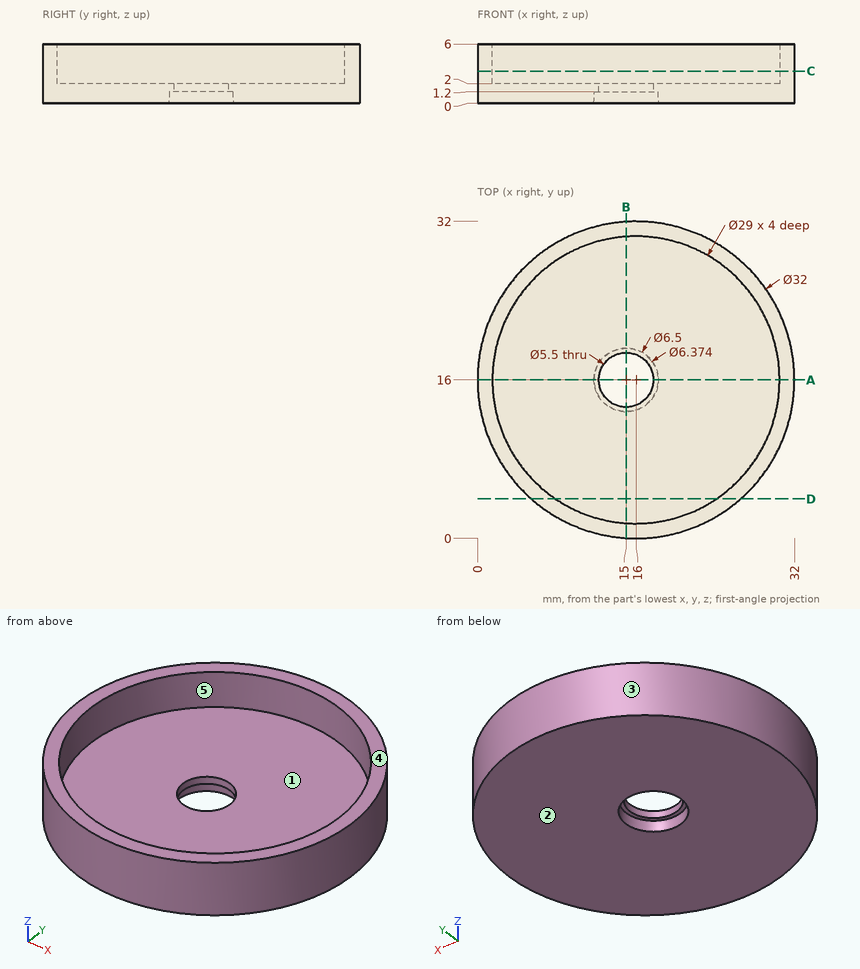
Print and shaded views of the part. All mm, measured from the part's lowest x, y and z. A direction names the side the tool comes from. Round coordinates to 2 decimals unless told otherwise and drop trailing zeros. Write each loop counter-clockwise with the first axis right and the second up, starting at its lowest first coordinate (ties: lowest second). Pieces come first, ordered by that corner, then holes. Notation, with made-up numbers: (75, 49.5) -> (93, 49.5) arc R24 cw to (93, 82.5) -> close; hole circle Ø11 at (-30, 53.25). An arc over 180 degrees is marked (long way). Answer in a Markdown table with one row per item. Add a question column.
Item 1: Drill centre lines: line 1 (Y direction, x = 16, z = 2.85); line 2 (Z direction, x = 22, y = 29); line 3 (X direction, y = 15, z = 0.95). Where is each one in solid material? Low to high. Write a range as from..to.
Item 2: Saw through at A-A, the plane y = 16. Write the cut outline in (x, z).
Item 3: Which spindle directions (+Z, -Z, +X, -X, +Y, -Y) get a long thin tool onto all of the face, cutting with end or side? Do the marked faces 4 and 5. Say none if no direction does.
Item 4: Drop flat-ended pins along their axis: pin 1 Ø12 at (x, y) = (5, 25) entering from +Z; pin 2 Ø1 at (x, y) = (14.5, 15) entering from -Z (3 decimals); pin 3 Ø1 at (x, z) = (26.5, 1) entering from +Y; pin 4 Ø1 at (x, y) = (16.5, 9.5) entering from +Z. Give the stop position or say it passes through.
Item 5: Mould opens along Y. For the marked faces 1, 2 and 3 say: pulls with the +Y half, pulls with the -Y half, needs draft (parallel to the pull), parting line crosses it, or undercut.
Item 6: Saw through at D-D, the plane y = 4. Write the cut outline in (x, z).
Item 7: Saw through at C-C, the plane z = 3.25. Write the cut outline in (x, y), then the cut area to 3 significant figures.
Item 8: Saw through at B-B, the plane x = 15. Write the cut outline in (y, z).
Findings below:
| question | item | result |
|---|---|---|
| 1 | line 1 | y = 0..1.5, 30.5..32 |
| 1 | line 2 | z = 0..2 |
| 1 | line 3 | x = 0.03..11.96, 18.04..31.97 |
| 2 | outline | (0, 0) -> (11.75, 0) -> (11.81, 1.2) -> (12.25, 1.2) -> (12.25, 2) -> (1.5, 2) -> (1.5, 6) -> (0, 6) -> close; (17.75, 1.2) -> (18.19, 1.2) -> (18.25, 0) -> (32, 0) -> (32, 6) -> (30.5, 6) -> (30.5, 2) -> (17.75, 2) -> close |
| 3 | face 4 | +Z, +X, -X, +Y, -Y |
| 3 | face 5 | +Z |
| 4 | pin 1 | stops at z = 6 |
| 4 | pin 2 | passes through |
| 4 | pin 3 | stops at y = 28.49 |
| 4 | pin 4 | stops at z = 2 |
| 5 | face 1 | undercut |
| 5 | face 2 | needs draft |
| 5 | face 3 | parting line crosses it |
| 6 | outline | (5.42, 0) -> (26.58, 0) -> (26.58, 6) -> (24.14, 6) -> (24.14, 2) -> (7.86, 2) -> (7.86, 6) -> (5.42, 6) -> close |
| 7 | outline | circle Ø32 at (16, 16); hole circle Ø29 at (16, 16) |
| 7 | area | 144 mm^2 |
| 8 | outline | (0.03, 0) -> (12.75, 0) -> (12.81, 1.2) -> (13.25, 1.2) -> (13.25, 2) -> (1.53, 2) -> (1.53, 6) -> (0.03, 6) -> close; (18.75, 1.2) -> (19.19, 1.2) -> (19.25, 0) -> (31.97, 0) -> (31.97, 6) -> (30.47, 6) -> (30.47, 2) -> (18.75, 2) -> close |
